Here's how the part is built. I have some questions about the finished solid (model axes, mm). A direction names the side the tool comes from. Round coordinates to 2 decimals unless told otherwise and drop trailing zeros. Write each loop counter-clockwise with the first axis right and the second up, starting at its lowest first coordinate (ties: lowest second). Pieces come first, ordered by that corner, then holes. Notation, with made-up numbers: M 40.5,54 L 50.5,54 A16 cw 50.5,82 Z; hole C 62.25,-2.5 d5. An arc over 180 degrees is marked long. Use one line per item in the form item = value. Start each with the question number.
Q1. We'd pull the mould along Y, two halves only. Please class faces 1 (the face through (-8, 0, 0)), 2 (the face through (-3.94, -0.07, 5.88)), 3 (the face through (-4.198, -11.923, -3.755)): +Y half, -Y half, draft (parallel to the pull), parting line (faces both ways), or undercut.
Q2. For faces 4 (the face through (19.211, 10.195, -2.264)), 5 (the face through (12.84, -1.604, 5.094)), 6 (the face through (0, 0, 7)), which set-ups out of +Z, -Z, +X, -X, +Y, -Y let a thin tool reach every point of the face, with its end or its side?
Q3. I want a section at A-A on x = 16.5. List the corners of the cut face in (y, z) for me, and give its area (3 significant figures).
Q4. I'm going to push flat-ended pins straight in: pin 1 Ø8 at (x, y) = (-3.5, -2.5) entering from +Z; pin 2 Ø1.5 at (x, y) = (12.5, -4.5) entering from -Z; pin 3 Ø1.6 at (y, z) = (0, 8) entering from -X; pin 4 Ø7 at (y, z) = (-1.5, 2) entering from +X. Where does each tip first touch, or does it pass through?
Q5. I need wall thicknesses on line 1 along Z through (x, y) = (-5.75, 0); line 2 along Z through (x, y) = (-5, -1); line 3 along Y through (x, z) = (-3, -7.5). Which ranges of each line are inside material? Lowest first, please. Write a range as from..to.
Solid Edge part; units mm, degrees
sketch "Sketch1" plane through (0, 0, 0) normal (0, -1, 0) x (1, 0, 0)
  line L0 (0, 10) -> (5, 10)
  line L1 (5, 10) -> (5, 5)
  line L2 (5, 5) -> (12.5, 5)
  line L3 (12.5, 5) -> (17.943, 10.443)
  line L4 (17.943, 10.443) -> (20.943, 10.443)
  line L5 (20.943, 10.443) -> (20.943, 8.443)
  line L6 (20.943, 8.443) -> (16.943, 0)
  line L7 (16.943, 0) -> (0, 0)
  line L8 (0, 0) -> (0, 10)
  dimension "D1" = 5
  dimension "D2" = 5
  dimension "D3" = 17.943
  dimension "D4" = 20.943
  dimension "D5" = 16.943
revolve "RevolvedProtrusion1" add sketch "Sketch1" angle 360 about axis through (-60, 0, 0) along (1, 0, 0)
sketch "Sketch2" plane through (0, 0, 0) normal (-1, 0, 0) x (0, -1, 0)
  circle A0 centre (0, 0) radius 12.5
extrude "Protrusion1" add sketch "Sketch2" along normal blind 8
hole "Bohrung_1" at (-8, 0, 7.5) direction (1, 0, 0) diameter 3.242 depth 8
hole "Hole1" at (-8, 0, -7.5) direction (1, 0, 0) diameter 3.242 depth 8
chamfer "Fase_1" distance 0.5 angle 45 1 edges at (0, 12.5, 0)
chamfer "Fase_2" distance 0.5 angle 45 1 edges at (5, 0, -10)
chamfer "Fase_3" distance 0.5 angle 45 1 edges at (20.943, 0, -10.443)
Reported:
q1.face_1 = draft
q1.face_2 = undercut
q1.face_3 = parting line
q2.face_4 = +X
q2.face_5 = none
q2.face_6 = -X
q3.outline = C 0,0 d18
q3.area = 254 mm^2
q4.pin_1 = 12.5
q4.pin_2 = -3.87
q4.pin_3 = 0
q4.pin_4 = 19.79
q5.line_1 = -12.5..-9.12, -5.88..5.88, 9.12..12.5
q5.line_2 = -12.46..-8.78, -6.22..6.22, 8.78..12.46
q5.line_3 = -10..-1.62, 1.62..10
